For this review, use the dimensioned drawing (mm, ordinates from the lowest corner) and the shaded views. Give positions to 0.01 mm unless a question says otherwise; leave off trailing zeros. Write each loop counter-clockwise with the first axis right and the second up, starting at its lowest first coordinate (ties: lowest second). Pieces come first, ordered by that corner, then holes. Notation, with made-up numbers: M 76,39.25 L 96,39.25 A26 cw 96,67.25 Z; hole C -33.5,-39 d9. An arc over 180 degrees is marked long. Answer in a Markdown table with one row per item.
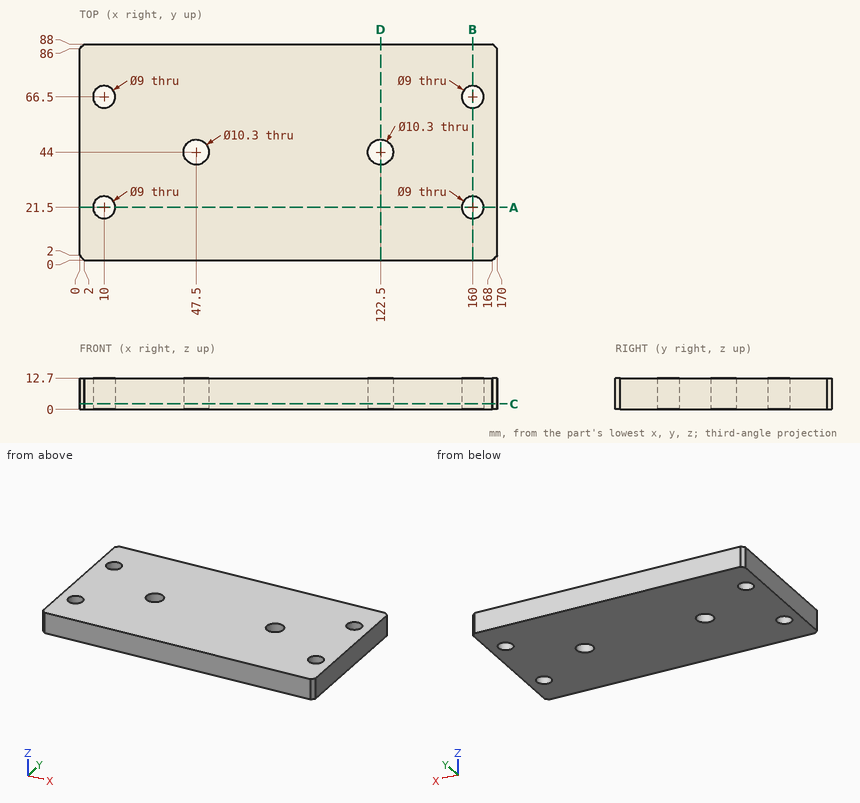
1) Add section A-A (y = 21.5). Write out the cut boundary in (x, z).
Geometry says:
| item | result |
|---|---|
| outline | M 0,0 L 5.5,0 L 5.5,12.7 L 0,12.7 Z; M 14.5,0 L 155.5,0 L 155.5,12.7 L 14.5,12.7 Z; M 164.5,0 L 170,0 L 170,12.7 L 164.5,12.7 Z |
2) Add section B-B (x = 160). Write out the cut boundary in (y, z).
Geometry says:
| item | result |
|---|---|
| outline | M 0,0 L 17,0 L 17,12.7 L 0,12.7 Z; M 26,0 L 62,0 L 62,12.7 L 26,12.7 Z; M 71,0 L 88,0 L 88,12.7 L 71,12.7 Z |
3) To check wall thickness, follow probe 1 along Y at (x, z) = (160, 9); probe 2 along Y at (x, z) = (47.5, 6); probe 3 along X at (y, z) = (20, 5.75). State the ranges of each line that lie inside material, in increasing order. Write a range as [from, to].
Geometry says:
| item | result |
|---|---|
| probe 1 | [0, 17], [26, 62], [71, 88] |
| probe 2 | [0, 38.85], [49.15, 88] |
| probe 3 | [0, 5.76], [14.24, 155.76], [164.24, 170] |
4) Add section D-D (x = 122.5). Write out the cut boundary in (y, z), and give its area (3 significant figures).
Geometry says:
| item | result |
|---|---|
| outline | M 0,0 L 38.85,0 L 38.85,12.7 L 0,12.7 Z; M 49.15,0 L 88,0 L 88,12.7 L 49.15,12.7 Z |
| area | 987 mm^2 |
5) Insertion check: P1, Ø16.5, axis at x = 47.5, y = 44, coming from the -Z side. The pin has a flat end and moves straight along its axis. Give the tip position at first contact, or say it passes through.
Geometry says:
| item | result |
|---|---|
| P1 | z = 0 |
6) Add section C-C (z = 2.25). Write out the cut boundary in (x, y).
Geometry says:
| item | result |
|---|---|
| outline | M 0,2 L 2,0 L 168,0 L 170,2 L 170,86 L 168,88 L 2,88 L 0,86 Z; hole C 10,21.5 d9; hole C 10,66.5 d9; hole C 47.5,44 d10.3; hole C 122.5,44 d10.3; hole C 160,21.5 d9; hole C 160,66.5 d9 |
